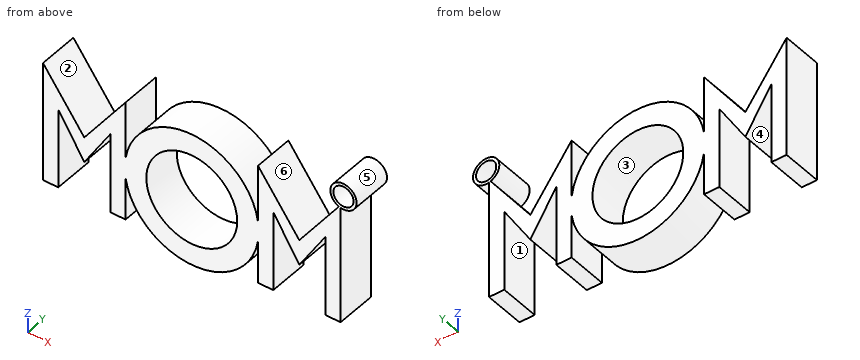
```python
from build123d import *

# Parameters (mm, degrees)
F0_R     = 14.4068230009
F0_R_2   = 3.2049597944
F1_DEPTH = 6.35


with BuildPart() as f1:
    # F0 (on Front) → F1 (new body, symmetric)
    with BuildSketch(Plane.XZ):
        with BuildLine():
            Line((-47.1492125925, -9.9419855554), (-42.3105131817, -9.9419855554))
            Line((-42.3105131817, -9.9419855554), (-42.3105131817, 15.4580144446))
            Line((-42.3105131817, 15.4580144446), (-34.0617353508, 2.3423101061))
            Line((-34.0617353508, 2.3423101061), (-25.8129575198, 15.4580144446))
            Line((-25.8129575198, 15.4580144446), (-25.8129575198, -9.9419855554))
            Line((-25.8129575198, -9.9419855554), (-20.974258109, -9.9419855554))
            Line((-20.974258109, -9.9419855554), (-20.974258109, 3.529483276))
            ThreePointArc((-20.974258109, 3.529483276), (-21.2326654511, 6.8319942802), (-20.974258109, 10.1345052844))
            Line((-20.974258109, 10.1345052844), (-20.974258109, 28.1580144446))
            Line((-20.974258109, 28.1580144446), (-34.0617353508, 10.3524101739))
            Line((-34.0617353508, 10.3524101739), (-47.1492125925, 28.1580144446))
            Line((-47.1492125925, 28.1580144446), (-47.1492125925, -9.9419855554))
        make_face()
        with BuildLine():
            ThreePointArc((21.0008528084, 9.9609339535), (0.0877984695, 28.0644782043), (-20.974258109, 10.1345052844))
            Line((-20.974258109, 10.1345052844), (-20.974258109, 3.529483276))
            ThreePointArc((-20.974258109, 3.529483276), (0.0877984695, -14.4004896439), (21.0008528084, 3.703054607))
            Line((21.0008528084, 3.703054607), (21.0008528084, 9.9609339535))
        make_face()
        with Locations((0, 6.8319942802)):
            Circle(F0_R, mode=Mode.SUBTRACT)
        with BuildLine():
            Line((-20.974258109, 3.529483276), (-20.974258109, 10.1345052844))
            ThreePointArc((-20.974258109, 10.1345052844), (-21.2326654511, 6.8319942802), (-20.974258109, 3.529483276))
        make_face()
        with BuildLine():
            Line((21.0008528084, 28.1580144446), (21.0008528084, 9.9609339535))
            ThreePointArc((21.0008528084, 9.9609339535), (21.1746329841, 8.4007517966), (21.2326654511, 6.8319942802))
            ThreePointArc((21.2326654511, 6.8319942802), (21.1746329841, 5.2632367639), (21.0008528084, 3.703054607))
            Line((21.0008528084, 3.703054607), (21.0008528084, -9.9419855554))
            Line((21.0008528084, -9.9419855554), (25.8395522192, -9.9419855554))
            Line((25.8395522192, -9.9419855554), (25.8395522192, 15.4580144446))
            Line((25.8395522192, 15.4580144446), (34.0883300501, 2.3423101061))
            Line((34.0883300501, 2.3423101061), (42.3371078811, 15.4580144446))
            Line((42.3371078811, 15.4580144446), (42.3371078811, -9.9419855554))
            Line((42.3371078811, -9.9419855554), (47.1758072919, -9.9419855554))
            Line((47.1758072919, -9.9419855554), (47.1758072919, 27.3316462631))
            ThreePointArc((47.1758072919, 27.3316462631), (46.923397405, 27.3967035148), (46.6755457316, 27.477405095))
            Line((46.6755457316, 27.477405095), (34.0883300501, 10.3524101739))
            Line((34.0883300501, 10.3524101739), (21.0008528084, 28.1580144446))
        make_face()
        with BuildLine():
            ThreePointArc((21.2326654511, 6.8319942802), (21.1746329841, 8.4007517966), (21.0008528084, 9.9609339535))
            Line((21.0008528084, 9.9609339535), (21.0008528084, 3.703054607))
            ThreePointArc((21.0008528084, 3.703054607), (21.1746329841, 5.2632367639), (21.2326654511, 6.8319942802))
        make_face()
        with BuildLine():
            ThreePointArc((52.2593864205, 31.3998535275), (45.6930221637, 34.8117766856), (46.6755457316, 27.477405095))
            Line((46.6755457316, 27.477405095), (47.1758072919, 28.1580144446))
            Line((47.1758072919, 28.1580144446), (47.1758072919, 27.3316462631))
            ThreePointArc((47.1758072919, 27.3316462631), (50.6950358132, 28.144354829), (52.2593864205, 31.3998535275))
        make_face()
        with Locations((48.0897761881, 31.3998535275)):
            Circle(F0_R_2, mode=Mode.SUBTRACT)
        with BuildLine():
            Line((47.1758072919, 28.1580144446), (46.6755457316, 27.477405095))
            ThreePointArc((46.6755457316, 27.477405095), (46.923397405, 27.3967035148), (47.1758072919, 27.3316462631))
            Line((47.1758072919, 27.3316462631), (47.1758072919, 28.1580144446))
        make_face()
    extrude(amount=F1_DEPTH, both=True)


solid = f1.part
```
Could you check a few things on this model? Use its own coordinates, in mm. Face numbers are marked on the shaded views. A direction names the side the tool comes from. Round coordinates to 2 decimals unless told otherwise and drop trailing zeros. Write each loop counter-clockwise with the first axis right and the second up, starting at its lowest first coordinate (ties: lowest second). Pieces come first, ordered by that corner, then holes. Notation, with made-up numbers: M 28,88 L 57,88 A27 cw 57,126 Z; hole C 60.25,-26 d3. An arc over 180 degrees is marked long. Write each question's results on one line, items separated by ' | '. Start each with the question number.
1. Imagine slicing it at A-A on x = 0. List the corners of the cut face in (y, z) for me.
2. On a 3-axis mill with a long thin cutter (end or side, diameter ignored), from which of +Z, -Z, +X, -X, +Y, -Y can I reach the whole of each face in a straight line? I mean the marked faces 1, 2 and 3. Say none if no direction works.
3. I need wall thicknesses on L1, parallel to X at y = 2, z = -1; L2, parallel to X at y = -4.5, z = 31.5; L3, parallel to X at y = -2.5, z = -6. Which ranges of each line are inside material? Lowest first, please. Write a range as from..to.
4. Thinking about a two-plate mould opening in Z: for the marked faces 4, 5 and 6, which applies, +Z half, -Z half, draft (parallel to the pull), parting line (faces both ways), or undercut?
5. Imagine slicing it at C-C on y = 5. List the corners of the cut face in (x, z) for me.
6. I'm going to push flat-ended pins straight in: pin 1 Ø1.5 at (x, y) = (-45, 2) entering from -Z; pin 2 Ø3 at (x, z) = (-7, -3.5) entering from +Y; pin 3 Ø7.5 at (x, z) = (48.09, 31.4) entering from -Y; pin 4 Ø2 at (y, z) = (3.5, 19.5) entering from +X. Where does each tip first touch, or does it pass through?
7. Imagine slicing it at D-D on z = 22.5. List the corners of the cut face in (x, y) for me.
8. Imagine slicing it at B-B on z = -3. List the corners of the cut face in (x, y) for me.
Result sheet:
1) outline: M -6.35,-14.4 L 6.35,-14.4 L 6.35,-7.57 L -6.35,-7.57 Z; M -6.35,21.24 L 6.35,21.24 L 6.35,28.06 L -6.35,28.06 Z
2) face 1: -Z, +Y, -Y | face 2: +Z, +Y, -Y | face 3: +Y, -Y
3) L1: x = -47.15..-42.31, -25.81..-20.97, -19.74..-12.09, 12.09..19.74, 21..25.84, 42.34..47.18 | L2: x = 43.92..44.89, 51.29..52.26 | L3: x = -47.15..-42.31, -25.81..-20.97, -16.92..-6.55, 6.55..16.92, 21..25.84, 42.34..47.18
4) face 4: -Z half | face 5: undercut | face 6: +Z half
5) outline: M -47.15,-9.94 L -42.31,-9.94 L -42.31,15.46 L -34.06,2.34 L -25.81,15.46 L -25.81,-9.94 L -20.97,-9.94 L -20.97,3.53 A21.23 ccw 21,3.7 L 21,-9.94 L 25.84,-9.94 L 25.84,15.46 L 34.09,2.34 L 42.34,15.46 L 42.34,-9.94 L 47.18,-9.94 L 47.18,27.33 A4.17 ccw long 46.68,27.48 L 34.09,10.35 L 21,28.16 L 21,9.96 A21.23 ccw -20.97,10.13 L -20.97,28.16 L -34.06,10.35 L -47.15,28.16 Z; hole C 0,6.83 d28.81; hole C 48.09,31.4 d6.41
6) pin 1: stops at z = -9.94 | pin 2: passes through | pin 3: stops at y = -6.35 | pin 4: stops at x = 47.18
7) outline: M -47.15,-6.35 L -42.99,-6.35 L -42.99,6.35 L -47.15,6.35 Z; M -25.13,-6.35 L -20.97,-6.35 L -20.97,6.35 L -25.13,6.35 Z; M -14.33,-6.35 L 14.33,-6.35 L 14.33,6.35 L -14.33,6.35 Z; M 21,-6.35 L 25.16,-6.35 L 25.16,6.35 L 21,6.35 Z; M 43.02,-6.35 L 47.18,-6.35 L 47.18,6.35 L 43.02,6.35 Z
8) outline: M -47.15,-6.35 L -42.31,-6.35 L -42.31,6.35 L -47.15,6.35 Z; M -25.81,-6.35 L -20.97,-6.35 L -20.97,6.35 L -25.81,6.35 Z; M -18.82,-6.35 L -10.53,-6.35 L -10.53,6.35 L -18.82,6.35 Z; M 10.53,-6.35 L 18.82,-6.35 L 18.82,6.35 L 10.53,6.35 Z; M 21,-6.35 L 25.84,-6.35 L 25.84,6.35 L 21,6.35 Z; M 42.34,-6.35 L 47.18,-6.35 L 47.18,6.35 L 42.34,6.35 Z
